Source: CAD feature listing. Evaluate the final solid. Frame: model axes, mm. A direction names the side the tool comes from. Give positions to 0.01 mm unless a question says otherwise; leave off trailing zeros. Order: outer loops, then holes, each group sorted by start corner. A loop starts at its lowest first (then second) coordinate and runs counter-clockwise, first axis right, second up. Notation, with made-up numbers: M 11,-5 L 28,-5 A18 cw 28,9 Z; hole C 11.25,-27 d3. An arc over 180 degrees is marked long. Answer in a Markdown table with one row per item. Add a question column.
(1) Section query A-A, the plane x = 668.5. Return loops of the section in (y, z), plus the area to 3 significant figures.
(2) Section query C-C, the plane y = -31.5. Return loops of the section in (x, z), plus the area to 3 significant figures.
(3) Material intervals for line 1 along X through (y, z) = (-226, 14.5); line 2 along X through (y, z) = (-103, 4.5); line 3 along Y through (x, z) = (155.5, 12.25), sorted ascending.
(4) Section query B-B, the plane z = 8.5. Return loops of the section in (x, y), plus the area to 3 significant figures.
(5) Pin query (flat end, axial travel): P1, Ø5.5, axis at x = 898.5, z = 12, coming from the -Y side; P2, Ø4, axis at y = -81.5, z = 10.5, coming from the -X side; P3, Ø1.5, axis at x = 761, z = 8.5, coming from the -Y side. Return the tip coordinate at first contact, or that it passes through.
(6) Mould query, pull axis Y, two halves, no side actions, for faces 1 (the face through (553, -72, 0)), 2 (the face through (711.3, -148.17, 9.42)), 3 (the face through (193.201, -157.584, 9.416)). Classes: pulls with the +Y half, pulls with the -Y half, needs draft (parallel to the pull), parting line crosses it, or undercut.
(7) Section query D-D, the plane x = 257. Return loops of the section in (y, z).
(8) Set-up query: faces 4 (the face through (217.96, -151.83, 9.42)), 5 (the face through (608, 0, 9)), 6 (the face through (694.6, -157.58, 9.42)). Return all of +Z, -Z, +X, -X, +Y, -Y with unobstructed straight access to the full face (end or side cutting, diameter ignored); none if empty.
from build123d import *

# Parameters (mm, degrees)
BOSS_EXTRUDE2_DEPTH = 19.1


with BuildPart() as part:
    # Sketch3 → Boss-Extrude2 (new body)
    with BuildSketch(Plane.XY):
        Polygon((391.889090758, -300), (408.110909242, -300), (600, -19.1), (791.889090758, -300), (808.110909242, -300), (1200, -19.1), (1200, 0), (0, 0), (0, -19.1), align=None)
        Polygon((32.785074333, -19.1), (576.868833396, -19.1), (398.027381063, -280.9), align=None, mode=Mode.SUBTRACT)
        Polygon((801.972618937, -280.9), (1167.214925667, -19.1), (623.131166604, -19.1), align=None, mode=Mode.SUBTRACT)
    extrude(amount=BOSS_EXTRUDE2_DEPTH)


solid = part.part
Values follow:
| question | item | result |
|---|---|---|
| 1 | outline | M -119.37,0 L -85.51,0 L -85.51,19.1 L -119.37,19.1 Z; M -19.1,0 L 0,0 L 0,19.1 L -19.1,19.1 Z |
| 1 | area | 1,010 mm² |
| 2 | outline | M 17.3,0 L 50.08,0 L 50.08,19.1 L 17.3,19.1 Z; M 568.4,0 L 591.53,0 L 591.53,19.1 L 568.4,19.1 Z; M 608.47,0 L 631.6,0 L 631.6,19.1 L 608.47,19.1 Z; M 1149.92,0 L 1182.7,0 L 1182.7,19.1 L 1149.92,19.1 Z |
| 2 | area | 2,140 mm² |
| 3 | line 1 | x = 288.65 to 321.44, 435.53 to 458.66, 741.34 to 764.47, 878.56 to 911.35 |
| 3 | line 2 | x = 117.05 to 149.84, 519.55 to 542.69, 657.31 to 680.45, 1050.16 to 1082.95 |
| 3 | line 3 | y = -130.56 to -107.06, -19.1 to 0 |
| 4 | outline | M 0,-19.1 L 391.89,-300 L 408.11,-300 L 600,-19.1 L 791.89,-300 L 808.11,-300 L 1200,-19.1 L 1200,0 L 0,0 Z; hole M 32.79,-19.1 L 398.03,-280.9 L 576.87,-19.1 Z; hole M 623.13,-19.1 L 801.97,-280.9 L 1167.21,-19.1 Z |
| 4 | area | 53,600 mm² |
| 5 | P1 | stops at y = -237.18 |
| 5 | P2 | stops at x = 84.27 |
| 5 | P3 | stops at y = -255.88 |
| 6 | face 1 | needs draft |
| 6 | face 2 | undercut |
| 6 | face 3 | pulls with the -Y half |
| 7 | outline | M -203.31,0 L -179.81,0 L -179.81,19.1 L -203.31,19.1 Z; M -19.1,0 L 0,0 L 0,19.1 L -19.1,19.1 Z |
| 8 | face 4 | +Z, -Z |
| 8 | face 5 | +Z, -Z, +X, -X, +Y |
| 8 | face 6 | +Z, -Z, -Y |
